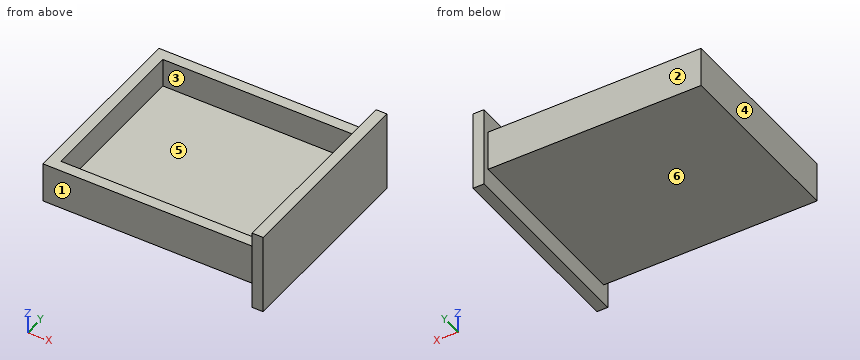
```python
from build123d import *

# Parameters (mm, degrees)
F0_W      = 370
F0_H      = 320
F1_DEPTH  = 70
F2_W      = 332
F2_H      = 282
F3_DEPTH  = 25
F3_FACE_W = 332
F3_FACE_H = 282
F4_DEPTH  = 11
F5_DEPTH  = 25
F6_W      = 342
F6_H      = 140
F6_W_2    = 320
F6_H_2    = 70
F7_DEPTH  = 19


with BuildPart() as f1:
    # F0 (on Top) → F1 (new body)
    with BuildSketch(Plane.XY):
        Rectangle(F0_W, F0_H)
    extrude(amount=F1_DEPTH)

    # F2 (on face) → F3 (cut)
    with BuildSketch(Plane.XY.offset(70)):
        Rectangle(F2_W, F2_H)
    extrude(amount=-F3_DEPTH, mode=Mode.SUBTRACT)

    # F3_face (on face) → F4 (join)
    with BuildSketch(Plane.XY.offset(45)):
        Rectangle(F3_FACE_W, F3_FACE_H)
    extrude(amount=-F4_DEPTH)

    # F3_face (on face) → F5 (cut)
    with BuildSketch(Plane.XY.offset(45)):
        Rectangle(F3_FACE_W, F3_FACE_H)
    extrude(amount=-F5_DEPTH, mode=Mode.SUBTRACT)

    # F6 (on face) → F7 (join)
    with BuildSketch(Plane.YZ.offset(185)):
        with Locations((0, 35)):
            Rectangle(F6_W, F6_H)
        with Locations((0, 35)):
            Rectangle(F6_W_2, F6_H_2, mode=Mode.SUBTRACT)
        with Locations((0, 35)):
            Rectangle(F6_W_2, F6_H_2)
    extrude(amount=F7_DEPTH)


solid = f1.part
```
The model under review builds one solid part; all positions refer to its coordinate system, in mm. Face numbers are marked on the shaded views. A direction names the side the tool comes from. Give positions to 0.01 mm unless a question says otherwise; leave off trailing zeros. Write each loop counter-clockwise with the first axis right and the second up, starting at its lowest first coordinate (ties: lowest second). Pieces come first, ordered by that corner, then holes. Notation, with made-up numbers: M -38.5,-1.5 L -25.5,-1.5 A30 ccw -25.5,34.5 Z; hole C -40,33.5 d3. An arc over 180 degrees is marked long. Write item = value, one per line. Start each with the question number.
Q1. Mouldability with a two-part tool opening along X and no side actions: class the marked faces 4, 5 and 6 as released by +X, released by -X, zero draft, split by the parting line, or undercut.
Q2. We need section D-D (y = 132). State the section outline as (x, z) points, plus the area to 3 significant figures.
Q3. We need section A-A (z = 7). State the section outline as (x, y) points, plus the area to 3 significant figures.
Q4. Machinability: for the marked faces 1, 2 and 3, which of the approach directions +Z, -Z, +X, -X, +Y, -Y give a long, thin tool a straight path to every point of the face, cutting with its end or side? Answer none if there is none.
Q5. We need section B-B (x = -7). State the section outline as (y, z) points, plus the area to 3 significant figures.
Q6. We need section C-C (z = 55). State the section outline as (x, y) points.
Q7. Clearance check with flat-ended pins moving along their axes: pin 1 (10 mm diameter, centred on x = -52.5, y = -50.5, fed in from -Z); pin 2 (10 mm diameter, centred on y = 31.5, z = 85, fed in from -X); pin 3 (21 mm diameter, centred on x = 10.5, z = 20.5, fed in from -Y). State where each tip first meets the part, or that it passes through.
Q8. For line 1 (Y direction, x = -143.5, z = 68); line 2 (X direction, y = 80.5, z = 24.5); line 3 (X direction, y = -64.5, z = -20), list the stretches that pass through material, from the lowest coordinate up.
Result set:
q1.face_4 = released by -X
q1.face_5 = undercut
q1.face_6 = zero draft
q2.outline = M -185,0 L 185,0 L 185,-35 L 204,-35 L 204,105 L 185,105 L 185,70 L 166,70 L 166,20 L -166,20 L -166,70 L -185,70 Z
q2.area = 12,000 mm2
q3.outline = M -185,-160 L 185,-160 L 185,-171 L 204,-171 L 204,171 L 185,171 L 185,160 L -185,160 Z
q3.area = 125,000 mm2
q4.face_1 = +Z, -Z, -X, -Y
q4.face_2 = +Z, -Z, -X, +Y
q4.face_3 = +Z
q5.outline = M -160,0 L 160,0 L 160,70 L 141,70 L 141,20 L -141,20 L -141,70 L -160,70 Z
q5.area = 8,300 mm2
q6.outline = M -185,-160 L 185,-160 L 185,-171 L 204,-171 L 204,171 L 185,171 L 185,160 L -185,160 Z; hole M -166,-141 L 166,-141 L 166,141 L -166,141 Z
q7.pin_1 = 0
q7.pin_2 = 185
q7.pin_3 = -160
q8.line_1 = -160 to -141, 141 to 160
q8.line_2 = -185 to -166, 166 to 204
q8.line_3 = 185 to 204
